from build123d import *

# Parameters (mm, degrees)
BOSS_EXTRUDE1_DEPTH = 3.175


with BuildPart() as part:
    # Sketch1 → Boss-Extrude1 (new body)
    with BuildSketch(Plane(origin=(0, 0, 0), x_dir=(1, 0, 0), z_dir=(0, 1, 0))):
        with BuildLine():
            Line((-6.35, 12.7), (6.35, 12.7))
            Line((6.35, 12.7), (6.35, 25.4))
            add(Edge.make_bspline(
                [(6.35, 56.328313115), (6.33277042, 33.531169368), (83.156548095, -1.798073983), (6.35, 25.4)],
                knots=[0, 0, 0, 0, 1, 1, 1, 1], degree=3))
            add(Edge.make_bspline(
                [(6.35, 76.947188524), (6.338513613, 61.749092693), (57.554365397, 38.196263793), (6.35, 56.328313115)],
                knots=[0, 0, 0, 0, 1, 1, 1, 1], degree=3))
            add(Edge.make_bspline(
                [(6.35, 90.693105464), (6.342342409, 80.561041577), (40.486243598, 64.859155643), (6.35, 76.947188524)],
                knots=[0, 0, 0, 0, 1, 1, 1, 1], degree=3))
            add(Edge.make_bspline(
                [(0, 101.6), (0.859116351, 99.501641609), (8.04674624, 94.542823282), (20.625145946, 84.684563188), (6.35, 90.693105464)],
                knots=[0, 0, 0, 0, 0.27708829, 1, 1, 1, 1], degree=3))
            add(Edge.make_bspline(
                [(0, 101.6), (-0.859116351, 99.501641609), (-8.04674624, 94.542823282), (-20.625145946, 84.684563188), (-6.35, 90.693105464)],
                knots=[0, 0, 0, 0, 0.27708829, 1, 1, 1, 1], degree=3))
            add(Edge.make_bspline(
                [(-6.35, 90.693105464), (-6.342342409, 80.561041577), (-40.486243598, 64.859155643), (-6.35, 76.947188524)],
                knots=[0, 0, 0, 0, 1, 1, 1, 1], degree=3))
            add(Edge.make_bspline(
                [(-6.35, 76.947188524), (-6.338513613, 61.749092693), (-57.554365397, 38.196263793), (-6.35, 56.328313115)],
                knots=[0, 0, 0, 0, 1, 1, 1, 1], degree=3))
            add(Edge.make_bspline(
                [(-6.35, 56.328313115), (-6.33277042, 33.531169368), (-83.156548095, -1.798073983), (-6.35, 25.4)],
                knots=[0, 0, 0, 0, 1, 1, 1, 1], degree=3))
            Line((-6.35, 25.4), (-6.35, 12.7))
        make_face()
    extrude(amount=-BOSS_EXTRUDE1_DEPTH)


solid = part.part
For this review, take the finished solid that the model builds, in its own axes (mm). A direction names the side the tool comes from. Round coordinates to 2 decimals unless told otherwise and drop trailing zeros. Use a Markdown table: item, result. Add a question column.
Item 1: To check wall thickness, follow line 1 along Z through (x, y) = (7.5, -1.55); line 2 along Z through (x, y) = (12.5, -2.7); line 3 along Z through (x, y) = (20.5, -1). State the ranges of each line that lie inside material, in increasing order.
Item 2: Tool access review of faces 3 (the flat face through (6.35, -2, -19)), 4 (the flat face through (0, -2, -12.7)): name each direction out of +Z, -Z, +X, -X, +Y, -Y from which nothing blocks a thin tool from reaching the whole face with its end or side.
Item 3: Mouldability with a two-part tool opening along X and no side actions: class faces 1 (the flat face through (0, -3.175, -50)), 2 (the flat face through (-6.35, -2, -19)) as released by +X, released by -X, zero draft, split by the parting line, or undercut.
Item 4: Add section A-A, the plane z = -20. State how many separate pieces and enclosed holes the cut face has, then the cut area to 3 significant figures.
Item 5: Insertion check: pin 1 (1 mm diameter, centred on x = 16, y = -0.5, fed in from +Z); pin 2 (1 mm diameter, centred on y = -2, z = -86, fed in from -X). Each pin has a flat end and moves straight along its axis. Give the tip position at first contact, or say it passes through.
Geometry results:
| question | item | result |
|---|---|---|
| 1 | line 1 | z = -94.72 to -90.22, -87.11 to -76.54, -72.64 to -55.92, -51.13 to -24.99 |
| 1 | line 2 | z = -90.64 to -88.5, -81.25 to -74.82, -65.85 to -54.18, -43.2 to -23.24 |
| 1 | line 3 | z = -74.27 to -72.59, -58.4 to -51.55, -34.79 to -20.52 |
| 2 | face 3 | +Z, +Y, -Y |
| 2 | face 4 | +Z, +X, -X, +Y, -Y |
| 3 | face 1 | zero draft |
| 3 | face 2 | undercut |
| 4 | separate pieces | 3 |
| 4 | enclosed holes | 0 |
| 4 | area | 139 mm² |
| 5 | pin 1 | stops at z = -21.86 |
| 5 | pin 2 | stops at x = -8.58 |
